Autodesk Inventor part; units mm, degrees
ref_plane "YZ Plane" through (0, 0, 0) normal (1, 0, 0) x (0, 1, 0)
ref_plane "XZ Plane" through (0, 0, 0) normal (0, 1, 0) x (-1, 0, 0)
ref_plane "XY Plane" through (0, 0, 0) normal (0, 0, 1) x (1, 0, 0)
sketch "Boceto1" plane through (0, 0, 0) normal (0, 1, 0) x (-1, 0, 0)
  line L0 (23.3407, 8.3801) -> (-1.6593, 8.3801)
  line L1 (-1.6593, 8.3801) -> (-1.6593, -16.6199)
  line L2 (-1.6593, -16.6199) -> (23.3407, -16.6199)
  line L3 (23.3407, -16.6199) -> (23.3407, 8.3801)
  circle A0 centre (1.3407, 3.3801) radius 1.7
  circle A1 centre (1.3407, -11.6199) radius 1.7
  circle A2 centre (12.3407, -11.6199) radius 1.7
  circle A3 centre (12.3407, 3.3801) radius 1.7
  line L4 (12.3407, -13.3199) -> (1.3407, -13.3199)
  line L5 (1.3407, -13.3199) -> (1.3407, -9.9199)
  line L6 (1.3407, -9.9199) -> (12.3407, -9.9199)
  line L7 (12.3407, -9.9199) -> (12.3407, -13.3199)
  line L8 (12.3407, 1.6801) -> (1.3407, 1.6801)
  line L9 (1.3407, 1.6801) -> (1.3407, 5.0801)
  line L10 (1.3407, 5.0801) -> (12.3407, 5.0801)
  line L11 (12.3407, 5.0801) -> (12.3407, 1.6801)
  point P0 (0, 0)
  point P1 (12.3407, 3.3801)
  point P2 (1.3407, -13.3199)
  point P3 (12.3407, 5.0801)
  point P4 (1.3407, 1.6801)
  dimension "d0" = 3.4
  dimension "d1" = 3
  dimension "d2" = 5
  dimension "d3" = 15
  dimension "d6" = 25
  dimension "d16" = 25
  dimension "d17" = 11
extrude "Extrusión1" add sketch "Boceto1" along normal blind 4
sketch "Boceto2" plane through (0, 4, 0) normal (0, 1, 0) x (1, 0, 0)
  line L0 (1.6593, 16.6199) -> (-23.3407, 16.6199)
  line L1 (-23.3407, -8.3801) -> (1.6593, -8.3801)
  line L2 (-23.3407, 16.6199) -> (-14.3407, 16.6199)
  line L3 (-14.3407, 16.6199) -> (-14.3407, -8.3801)
  line L4 (-14.3407, -8.3801) -> (-23.3407, -8.3801)
  line L5 (-23.3407, -8.3801) -> (-23.3407, 16.6199)
  point P0 (0, 0)
  point P1 (-14.3407, 16.6199)
  dimension "d7" = 9
extrude "Extrusión2" add sketch "Boceto2" against normal blind 7
sketch "Boceto5" plane through (0, -3, 0) normal (0, -1, 0) x (1, 0, 0)
  line L0 (-14.3407, 8.3801) -> (-23.3407, 8.3801)
  line L1 (-23.3407, 8.3801) -> (-14.3407, 8.3801)
  line L2 (-14.3407, 8.3801) -> (-14.3407, 14.3801)
  line L3 (-14.3407, 14.3801) -> (-23.3407, 14.3801)
  line L4 (-23.3407, 14.3801) -> (-23.3407, 8.3801)
  line L5 (-14.3407, -16.6199) -> (-14.3407, 8.3801)
  point P0 (0, 0)
  dimension "d24" = 6
extrude "Extrusión5" add sketch "Boceto5" against normal up to surface (7 mm away)
fillet "Empalme2" radius 5 1 edges at (-14.3407, 2, 8.3801)
sketch "Boceto3" plane through (0, -3, 0) normal (0, -1, 0) x (1, 0, 0)
  circle A0 centre (-17.3407, 9.8801) radius 1.2
  circle A1 centre (-17.3407, 0.3801) radius 1.2
  line L0 (-14.3407, -16.6199) -> (-14.3407, 8.3801)
  line L1 (-23.3407, -16.6199) -> (-14.3407, -16.6199)
  line L2 (-23.3407, 14.3801) -> (-23.3407, -16.6199)
  point P0 (0, 0)
  dimension "d10" = 2.4
  dimension "d11" = 9.5
  dimension "d19" = 17
  dimension "d30" = 6
extrude "Extrusión3" cut sketch "Boceto3" against normal through all
sketch "Boceto4" plane through (0, 4, 0) normal (0, 1, 0) x (1, 0, 0)
  circle A0 centre (-17.3407, -9.8801) radius 1.2
  circle A1 centre (-17.3407, -9.8801) radius 2.15
  line L0 (-17.3407, -12.3627) -> (-19.4907, -11.1214)
  line L1 (-19.4907, -11.1214) -> (-19.4907, -8.6388)
  line L2 (-19.4907, -8.6388) -> (-17.3407, -7.3975)
  line L3 (-17.3407, -7.3975) -> (-15.1907, -8.6388)
  line L4 (-15.1907, -8.6388) -> (-15.1907, -11.1214)
  line L5 (-15.1907, -11.1214) -> (-17.3407, -12.3627)
  circle A2 centre (-17.3407, -0.3801) radius 1.2
  circle A3 centre (-17.3407, -0.3801) radius 2.15
  line L6 (-17.3407, 2.1025) -> (-15.1907, 0.8612)
  line L7 (-15.1907, 0.8612) -> (-15.1907, -1.6214)
  line L8 (-15.1907, -1.6214) -> (-17.3407, -2.8627)
  line L9 (-17.3407, -2.8627) -> (-19.4907, -1.6214)
  line L10 (-19.4907, -1.6214) -> (-19.4907, 0.8612)
  line L11 (-19.4907, 0.8612) -> (-17.3407, 2.1025)
  point P0 (0, 0)
  dimension "d29" = 4.3
extrude "Extrusión4" cut sketch "Boceto4" against normal blind 5 contours A0 | A1 | L4 L5 A1 | A1 L3 L4 | A1 L2 L3 | L5 L0 A1 | A1 L1 L2 | L0 L1 A1 | A2 | A3 | L7 L8 A3 | A3 L6 L7 | A3 L11 L6 | L8 L9 A3 | A3 L10 L11 | L9 L10 A3
fillet "Empalme3" radius 3 4 edges at (-23.3407, 0.5, 14.3801) (-23.3407, 0.5, -16.6199) (1.6593, 2, 8.3801) (1.6593, 2, -16.6199)
sketch "Boceto6" plane through (0, 0, 0) normal (0, -1, 0) x (1, 0, 0)
  point P0 (0, 0)
sketch "Boceto7" plane through (0, -3, 0) normal (0, -1, 0) x (1, 0, 0)
  arc A0 (-12.3407, 5.0801) -> (-12.3407, 1.6801) centre (-12.3407, 3.3801) ccw
  circle A1 centre (-12.3407, 3.3801) radius 3
  arc A2 (-12.3407, -9.9199) -> (-12.3407, -13.3199) centre (-12.3407, -11.6199) ccw
  circle A3 centre (-12.3407, -11.6199) radius 3
  point P0 (0, 0)
  dimension "d31" = 6
  dimension "d32" = 6
extrude "Extrusión6" cut sketch "Boceto7" against normal up to surface (3 mm away)
properties part number "shoulder endstop support"
Can you work these out from the model? Positions are in its coordinate system, mm. A direction names the side the tool comes from. Round coordinates to 2 decimals unless told otherwise and drop trailing zeros. Order: outer loops, then holes, each group sorted by start corner. A loop starts at its lowest first (then second) coordinate and runs counter-clockwise, first axis right, second up. Notation, with made-up numbers: (38, 63.25) - (63, 63.25) arc R17 cw to (63, 83.25) - close; hole circle Ø9 at (87.5, 83.25). An arc over 180 degrees is marked (long way). Answer in a Markdown table with one row per item.
(1) Suppose I cut it at A-A, the plane x = -4.5. Please give me the cut outline in (y, z), plus the area to 3 significant figures.
From the geometry:
| item | result |
|---|---|
| outline | (0, -16.62) - (4, -16.62) - (4, -13.32) - (0, -13.32) - close; (0, -9.92) - (4, -9.92) - (4, 1.68) - (0, 1.68) - close; (0, 5.08) - (4, 5.08) - (4, 8.38) - (0, 8.38) - close |
| area | 72.8 mm2 |
(2) Suppose I cut it at D-D, the plane y = -2. Please give me the cut outline in (x, z), plus the area to 3 significant figures.
From the geometry:
| item | result |
|---|---|
| outline | (-23.34, -13.62) arc R3 ccw to (-20.34, -16.62) - (-14.34, -16.62) - (-14.34, -13.86) arc R3 cw to (-14.34, -9.38) - (-14.34, 1.14) arc R3 cw to (-14.34, 5.62) - (-14.34, 14.38) - (-20.34, 14.38) arc R3 ccw to (-23.34, 11.38) - close; hole circle Ø2.4 at (-17.34, 0.38); hole circle Ø2.4 at (-17.34, 9.88) |
| area | 260 mm2 |
(3) Suppose I cut it at C-C, the plane z = 4. Please give me the cut outline in (x, y), plus the area to 3 significant figures.
From the geometry:
| item | result |
|---|---|
| outline | (-23.34, -3) - (-15.28, -3) - (-15.28, 0) - (-13.92, 0) - (-13.92, 4) - (-23.34, 4) - close; (0.24, 0) - (1.66, 0) - (1.66, 4) - (0.24, 4) - close |
| area | 67.5 mm2 |
(4) Please list where these lines run through material, in increasing order: L1, parallel to Z at x = -1.5, y = 2.5; L2, parallel to Z at x = -15.5, y = 2; L3, parallel to Y at x = -8.5, z = 7.5. Write a range as from..to.
From the geometry:
| item | result |
|---|---|
| L1 | z = -16.62..-13.32, -9.92..1.68, 5.08..8.38 |
| L2 | z = -16.62..-1.04, 1.8..8.46, 11.3..14.38 |
| L3 | y = 0..4 |
(5) If we mould it in two halves opening along X, with no side actions, what happens to faces 1 (the face through (-22.485, 0.549, 13.478)), 2 (the face through (-15.34, -1.52, -11.58)), 3 (the face through (-16.251, 1.535, 11.733)), 4 (the face through (-16.3, 1.5, 8))? For each: released by +X, released by -X, zero draft, split by the parting line, or undercut.
From the geometry:
| item | result |
|---|---|
| face 1 | released by -X |
| face 2 | released by +X |
| face 3 | undercut |
| face 4 | undercut |
(6) Suppose I cut it at B-B, the plane y = 0.5. Count the separate pieces of the cut face and the enclosed holes in it, plus the area to 3 significant figures.
From the geometry:
| item | result |
|---|---|
| separate pieces | 1 |
| enclosed holes | 4 |
| area | 552 mm2 |
(7) For P1, Ø1, axis at x = -7.5, z = -12, coming from the +Y side; P2, Ø4, axis at x = -17.34, z = 9.88, coming from the +Y side; P3, Ø2, axis at y = 2, z = 11, coming from the +X side; P4, Ø1, axis at x = -9, y = 0.5, coming from the +Z side, each with a flat end and sliding along its axis, tell me the tip position at first contact or that it passes through.
From the geometry:
| item | result |
|---|---|
| P1 | passes through |
| P2 | stops at y = -1 |
| P3 | stops at x = -13.03 |
| P4 | stops at z = 8.38 |
(8) Which directions (+Z, -Z, +X, -X, +Y, -Y) give clear straight access to the entire face, cutting with the end or side of a thin tool? Please do faces 5 (the face through (-18, -1, -1)), 6 (the face through (-14.341, -2, -15)), 7 (the face through (0.36, 1.97, -11.66)).
From the geometry:
| item | result |
|---|---|
| face 5 | +Y |
| face 6 | +Z, -Z, +X, -Y |
| face 7 | +Y, -Y |
